from build123d import *

# Parameters (mm, degrees)
SKETCH1_W           = 150
SKETCH1_H           = 120
BOSS_EXTRUDE1_DEPTH = 5
SKETCH2_R           = 3.05
CUT_EXTRUDE1_DEPTH  = 10
FILLET1_R           = 3


with BuildPart() as part:
    # Sketch1 → Boss-Extrude1 (new body)
    with BuildSketch(Plane(origin=(0, 0, 0), x_dir=(1, 0, 0), z_dir=(0, 1, 0))):
        Rectangle(SKETCH1_W, SKETCH1_H)
    extrude(amount=BOSS_EXTRUDE1_DEPTH)

    # Sketch2 → Cut-Extrude1 (cut)
    with BuildSketch(Plane(origin=(0, 5, 0), x_dir=(1, 0, 0), z_dir=(0, 1, 0))):
        with Locations(Location((-30, 30, 0), (0, 0, 270))):
            Circle(SKETCH2_R)
        with Locations(Location((30, 30, 0), (0, 0, 270))):
            Circle(SKETCH2_R)
        with Locations(Location((30, -30, 0), (0, 0, 270))):
            Circle(SKETCH2_R)
        with Locations(Location((-30, -30, 0), (0, 0, 270))):
            Circle(SKETCH2_R)
        with Locations(Location((-65, 50, 0), (0, 0, 270))):
            Circle(SKETCH2_R)
        with Locations(Location((65, 50, 0), (0, 0, 270))):
            Circle(SKETCH2_R)
        with Locations(Location((-65, -50, 0), (0, 0, 270))):
            Circle(SKETCH2_R)
        with Locations(Location((65, -50, 0), (0, 0, 270))):
            Circle(SKETCH2_R)
    extrude(amount=-CUT_EXTRUDE1_DEPTH, mode=Mode.SUBTRACT)

    # Fillet1
    fillet1_edges = [part.edges().sort_by_distance(p)[0] for p in [
        (75, 2.5, 60),
        (-75, 2.5, 60),
        (-75, 2.5, -60),
        (75, 2.5, -60),
    ]]
    fillet(fillet1_edges, radius=FILLET1_R)


solid = part.part
Source: CAD feature listing. Evaluate the final solid. Frame: model axes, mm. Give positions to 0.01 mm unless a question says otherwise; leave off trailing zeros. Write each loop counter-clockwise with the first axis right and the second up, starting at its lowest first coordinate (ties: lowest second). Pieces come first, ordered by that corner, then holes. Notation, with made-up numbers: M 71,-31.75 L 114,-31.75 A25 ccw 114,-19.75 Z; hole C 65.25,-19 d9. An arc over 180 degrees is marked long. Return JSON: item names as keys, results as strings. Group by question number.
1) Pin query (flat end, axial travel): P1, Ø3.5, axis at x = -65, z = 50, coming from the +Y side. Return the tip coordinate at first contact, or that it passes through.
2) Cut plane B-B, the plane z = 50. Output: boundary loops of the cut face in (x, y).
3) Cut plane A-A, the plane x = -65. Output: boundary loops of the cut face in (y, z).
4) Pull-direction query (Z, two-part tool) for faces 1 (the face through (-74.14, 2.54, 59.1)), 2 (the face through (-74.14, 2.54, -59.1)), 3 (the face through (-32.706, 2.535, 31.407)), 4 (the face through (-75, 2, 1)); classes: pulls with the +Z half, pulls with the -Z half, needs draft (parallel to the pull), parting line crosses it, or undercut.
5) Material intervals for line 1 along X through (y, z) = (1.4, 50); line 2 along X through (y, z) = (2.05, -30), sorted ascending. Write a range as [from, to].
Recorded:
{
 "1": {"P1": "passes through"},
 "2": {"outline": "M -75,0 L -68.05,0 L -68.05,5 L -75,5 Z; M -61.95,0 L 61.95,0 L 61.95,5 L -61.95,5 Z; M 68.05,0 L 75,0 L 75,5 L 68.05,5 Z"},
 "3": {"outline": "M 0,-60 L 5,-60 L 5,-53.05 L 0,-53.05 Z; M 0,-46.95 L 5,-46.95 L 5,46.95 L 0,46.95 Z; M 0,53.05 L 5,53.05 L 5,60 L 0,60 Z"},
 "4": {"face 1": "pulls with the +Z half", "face 2": "pulls with the -Z half", "face 3": "undercut", "face 4": "needs draft"},
 "5": {"line 1": "x = [-75, -68.05], [-61.95, 61.95], [68.05, 75]", "line 2": "x = [-75, -33.05], [-26.95, 26.95], [33.05, 75]"}
}
